```python
from build123d import *

# Parameters (mm, degrees)
SKETCH1_W           = 177.8
SKETCH1_H           = 76.2
BOSS_EXTRUDE1_DEPTH = 165.1
SKETCH2_W           = 50.8
SKETCH2_H           = 25.4
CUT_EXTRUDE1_DEPTH  = 15.24
SKETCH3_W           = 177.8
SKETCH3_H           = 76.2
SKETCH3_W_2         = 175.26
SKETCH3_H_2         = 73.66
CUT_EXTRUDE2_DEPTH  = 1.27


with BuildPart() as part:
    # Sketch1 → Boss-Extrude1 (new body)
    with BuildSketch(Plane(origin=(0, 0, 0), x_dir=(1, 0, 0), z_dir=(0, 1, 0))):
        with Locations((88.9, 38.1)):
            Rectangle(SKETCH1_W, SKETCH1_H)
    extrude(amount=BOSS_EXTRUDE1_DEPTH)

    # Sketch2 → Cut-Extrude1 (cut)
    with BuildSketch(Plane(origin=(0, 165.1, 0), x_dir=(1, 0, 0), z_dir=(0, 1, 0))):
        with Locations((25.4, 12.7)):
            Rectangle(SKETCH2_W, SKETCH2_H)
        with Locations((152.4, 12.7)):
            Rectangle(SKETCH2_W, SKETCH2_H)
    extrude(amount=-CUT_EXTRUDE1_DEPTH, mode=Mode.SUBTRACT)

    # Sketch3 → Cut-Extrude2 (cut)
    with BuildSketch(Plane(origin=(0, 139.7, 0), x_dir=(1, 0, 0), z_dir=(0, 1, 0))):
        with Locations((88.9, 38.1)):
            Rectangle(SKETCH3_W, SKETCH3_H)
        with Locations((88.9, 38.1)):
            Rectangle(SKETCH3_W_2, SKETCH3_H_2, mode=Mode.SUBTRACT)
    extrude(amount=-CUT_EXTRUDE2_DEPTH, mode=Mode.SUBTRACT)


solid = part.part
```
Model file for the job. Use its own axes, mm. A direction names the side the tool comes from. Coordinates: 2 decimals unless noted, no trailing zeros. Order: outer loops, then holes, each group sorted by start corner. A loop starts at its lowest first (then second) coordinate and runs counter-clockwise, first axis right, second up. Notation, with made-up numbers: (-10, -8.5) - (35, -8.5) arc R20 cw to (35, 26.5) - close; hole circle Ø8 at (-35.75, 64.5). An arc over 180 degrees is marked (long way). Return JSON: item names as keys, results as strings. Group by question number.
1) Flat gauge pins, fed straight in: P1, Ø12.5, axis at x = 22, z = -7.5, coming from the +Y side; P2, Ø7.5, axis at x = 16.5, y = 160, coming from the +Z side; P3, Ø0.6, axis at y = 139, z = -37, coming from the +X side. Where does each tip first touch, or does it go through?
2) Probe line 1 (X direction, y = 139, z = -59); line 2 (Y direction, x = 13, z = -14). List the from-to ranges inside material, lowest first. Write a range as from..to.
3) Saw through at A-A, the plane x = 30.5. Write the cut outline in (y, z), plus the area to 3 significant figures.
4) Tool access for faces 1 (the flat face through (25, 149.86, -13)), 2 (the flat face through (0, 68, -38)), 3 (the flat face through (152, 149.86, -13)): list every direction of +Z, -Z, +X, -X, +Y, -Y with a clear straight run to the whole face (end or side of a thin tool).
5) Saw through at B-B, the plane z = -19.5. Write the cut outline in (x, y).
Values found:
{
 "1": {"P1": "stops at y = 149.86", "P2": "stops at z = -25.4", "P3": "stops at x = 176.53"},
 "2": {"line 1": "x = 1.27..176.53", "line 2": "y = 0..149.86"},
 "3": {"outline": "(0, -76.2) - (138.43, -76.2) - (138.43, -74.93) - (139.7, -74.93) - (139.7, -76.2) - (165.1, -76.2) - (165.1, -25.4) - (149.86, -25.4) - (149.86, 0) - (139.7, 0) - (139.7, -1.27) - (138.43, -1.27) - (138.43, 0) - (0, 0) - close", "area": "12,200 mm²"},
 "4": {"face 1": "+Z, -X, +Y", "face 2": "+Z, -Z, -X, +Y, -Y", "face 3": "+Z, +X, +Y"},
 "5": {"outline": "(0, 0) - (177.8, 0) - (177.8, 138.43) - (176.53, 138.43) - (176.53, 139.7) - (177.8, 139.7) - (177.8, 149.86) - (127, 149.86) - (127, 165.1) - (50.8, 165.1) - (50.8, 149.86) - (0, 149.86) - (0, 139.7) - (1.27, 139.7) - (1.27, 138.43) - (0, 138.43) - close"}
}
